CAD build for the part. Positions are in the model's coordinates, mm. A direction names the side the tool comes from. Give positions to 0.01 mm unless a question says otherwise; leave off trailing zeros. Loops run counter-clockwise (first coordinate to the right, second up) from the corner with the lowest first, then second, coordinate; pieces in that order, holes last.
Item 1: Probe probe 1 along Y at (x, z) = (-42.5, -12.5); probe 2 along Z at (x, y) = (5.5, 18.5). List the from-to ranges inside material, lowest first.
Item 2: Saw through at B-B on z = -12.5. Give the cut face in (x, y), plus the area to 3 significant figures.
Item 3: Saw through at A-A on y = 0. Give the cut face in (x, z).
Item 4: Mould opens along Z. For faces 1 (the flat face through (43, -12.5, -12)), 2 (the flat face through (-1, 0, 150)), 3 (the cylindrical face through (42, 0, -15)) say: released by +Z, released by -Z, zero draft, split by the parting line, or undercut.
Item 5: Saw through at D-D on y = 10. Give the cut face in (x, z).
Item 6: Which spindle directions (+Z, -Z, +X, -X, +Y, -Y) get a long thin tool onto all of the face, cutting with end or side? Do faces 4 (the flat face through (-1, 29, 74)), 5 (the flat face through (35, -0.2, -9.5)), 6 (the flat face through (-42, -12.5, -12)), 7 (the flat face through (43, 12.5, -12)). Say none if no direction does.
Item 7: Saw through at C-C on x = -4. Give the cut face in (y, z).
Item 8: Drop flat-ended pins along their axis: P1, Ø4.5, axis at y = 0, z = -12.5, coming from the +X side; P2, Ø2, axis at x = -18.5, y = 10.5, coming from the -Z side; P3, Ø7.5, axis at x = -45, z = -8.5, coming from the +Y side; P4, Ø16.5, axis at x = 39.5, z = -10.5, coming from the -Y side. Give the stop position or say it passes through.
from build123d import *

# Parameters (mm, degrees)
SKETCH2_W           = 100
SKETCH2_H           = 58
BOSS_EXTRUDE1_DEPTH = 150
SKETCH3_W           = 15
SKETCH3_H           = 25
BOSS_EXTRUDE2_DEPTH = 25
CUT_EXTRUDE1_REACH  = 184.595
SKETCH4_R           = 2.5


with BuildPart() as part:
    # Sketch2 → Boss-Extrude1 (new body)
    with BuildSketch(Plane.XY):
        Rectangle(SKETCH2_W, SKETCH2_H)
    extrude(amount=BOSS_EXTRUDE1_DEPTH)

    # Sketch3 → Boss-Extrude2 (add)
    with BuildSketch(Plane(origin=(0, 0, 0), x_dir=(-1, 0, 0), z_dir=(0, 0, -1))):
        with Locations((42.5, 0)):
            Rectangle(SKETCH3_W, SKETCH3_H)
        with Locations((-42.5, 0)):
            Rectangle(SKETCH3_W, SKETCH3_H)
    extrude(amount=BOSS_EXTRUDE2_DEPTH)

    # Cut-Extrude1: up to this face of the body (flat: up to its plane)
    cut_extrude1_end = Plane(part.part.faces().sort_by_distance((50, 0, 69.13538874))[0])
    # Sketch4 → Cut-Extrude1 (cut, up to the picked face)
    with BuildSketch(Plane.ZY.offset(50), mode=Mode.PRIVATE) as cut_extrude1_sk1:
        with Locations((-12.5, 0)):
            Circle(SKETCH4_R)
    cut_extrude1_tool1 = split(extrude(cut_extrude1_sk1.sketch, amount=-CUT_EXTRUDE1_REACH, mode=Mode.PRIVATE), bisect_by=cut_extrude1_end, keep=Keep.BOTH, mode=Mode.PRIVATE)
    add(cut_extrude1_tool1.solids().sort_by(Axis((-50, 0, -12.5), (1, 0, 0)))[0], mode=Mode.SUBTRACT)


solid = part.part
Results below:
1. probe 1: y = -12.5 to -2.5, 2.5 to 12.5
1. probe 2: z = 0 to 150
2. outline: (-50, -12.5) - (-35, -12.5) - (-35, -2.5) - (-50, -2.5) - close; (-50, 2.5) - (-35, 2.5) - (-35, 12.5) - (-50, 12.5) - close; (35, -12.5) - (50, -12.5) - (50, -2.5) - (35, -2.5) - close; (35, 2.5) - (50, 2.5) - (50, 12.5) - (35, 12.5) - close
2. area: 600 mm2
3. outline: (-50, -25) - (-35, -25) - (-35, -15) - (-50, -15) - close; (-50, -10) - (-35, -10) - (-35, 0) - (35, 0) - (35, -10) - (50, -10) - (50, 150) - (-50, 150) - close; (35, -25) - (50, -25) - (50, -15) - (35, -15) - close
4. face 1: zero draft
4. face 2: released by +Z
4. face 3: undercut
5. outline: (-50, -25) - (-35, -25) - (-35, 0) - (35, 0) - (35, -25) - (50, -25) - (50, 150) - (-50, 150) - close
6. face 4: +Z, -Z, +X, -X, +Y
6. face 5: -Z, +Y, -Y
6. face 6: -Z, +X, -X, -Y
6. face 7: -Z, +X, -X, +Y
7. outline: (-29, 0) - (29, 0) - (29, 150) - (-29, 150) - close
8. P1: passes through
8. P2: stops at z = 0
8. P3: stops at y = 12.5
8. P4: stops at y = -12.5
